Work out the finished part from the listing and answer in its coordinate system (mm). A direction names the side the tool comes from. Coordinates: 2 decimals unless noted, no trailing zeros. Write each loop counter-clockwise with the first axis right and the second up, starting at its lowest first coordinate (ties: lowest second). Pieces come first, ordered by that corner, then holes. Notation, with made-up numbers: (79, -37) - (104, -37) arc R35 cw to (104, -3) - close; hole circle Ø10 at (35, 8.5). An arc over 180 degrees is marked (long way). Use a Markdown table: item, result. Add a question column.
(1) The part is cut by section A-A, the plane z = 3. Give the vertices of the cut face in (x, y), then the cut area to 3 significant figures.
(2) Find the intervals of material crossed by line 1 (X direction, y = 13.5, z = 1.75); line 2 (Y direction, x = -61, z = 24.5); line 3 (Y direction, x = -69, z = 12.5), in increasing order. Write a range as from..to.
(3) A tool of negligible diameter and unlimited length cuts with its end or side. For faces 1 (the face through (-38.98, 23, 13)), 2 (the face through (-1, -95.177, 13)), 3 (the face through (38.98, 23, 13)), from which of +Z, -Z, +X, -X, +Y, -Y can it reach the whole face along a straight path? Write none if from no direction.
(4) The part is cut by section B-B, the plane y = 37.5. Give the vertices of the cut face in (x, z), then the cut area to 3 significant figures.
(5) Given pin 1 Ø7.5 at (y, z) = (25.5, 17) entering from -X; pin 2 Ø7.5 at (y, z) = (7, 14.5) entering from +X, each flat-ended and moving along its own axis, determine where each tip first touches the part or whether it passes through.
(6) The part is cut by section C-C, the plane y = -72. Give the vertices of the cut face in (x, z), then the cut area to 3 significant figures.
from build123d import *

# Parameters (mm, degrees)
F0_W     = 77.960826
F0_H     = 91.74003
F1_DEPTH = 25.4
F2_DEPTH = 25.4


with BuildPart() as f1:
    # F0 (on Top) → F1 (new body)
    with BuildSketch(Plane.XY):
        with Locations((0, 23.481315)):
            Rectangle(F0_W, F0_H)
    extrude(amount=F1_DEPTH)

    # F0 (on Top) → F2 (join)
    with BuildSketch(Plane.XY):
        Polygon((-76.578632, -95.176995), (76.578632, -95.176995), (38.980413, -22.3887), (-38.980413, -22.3887), align=None)
    extrude(amount=F2_DEPTH)


solid = f1.part
Model answer:
| question | item | result |
|---|---|---|
| 1 | outline | (-76.58, -95.18) - (76.58, -95.18) - (38.98, -22.39) - (38.98, 69.35) - (-38.98, 69.35) - (-38.98, -22.39) - close |
| 1 | area | 15,600 mm^2 |
| 2 | line 1 | -38.98..38.98 |
| 2 | line 2 | -95.18..-65.02 |
| 2 | line 3 | -95.18..-80.51 |
| 3 | face 1 | +Z, -Z, -X, +Y |
| 3 | face 2 | +Z, -Z, +X, -X, -Y |
| 3 | face 3 | +Z, -Z, +X, +Y |
| 4 | outline | (-38.98, 0) - (38.98, 0) - (38.98, 25.4) - (-38.98, 25.4) - close |
| 4 | area | 1,980 mm^2 |
| 5 | pin 1 | x = -38.98 |
| 5 | pin 2 | x = 38.98 |
| 6 | outline | (-64.61, 0) - (64.61, 0) - (64.61, 25.4) - (-64.61, 25.4) - close |
| 6 | area | 3,280 mm^2 |
